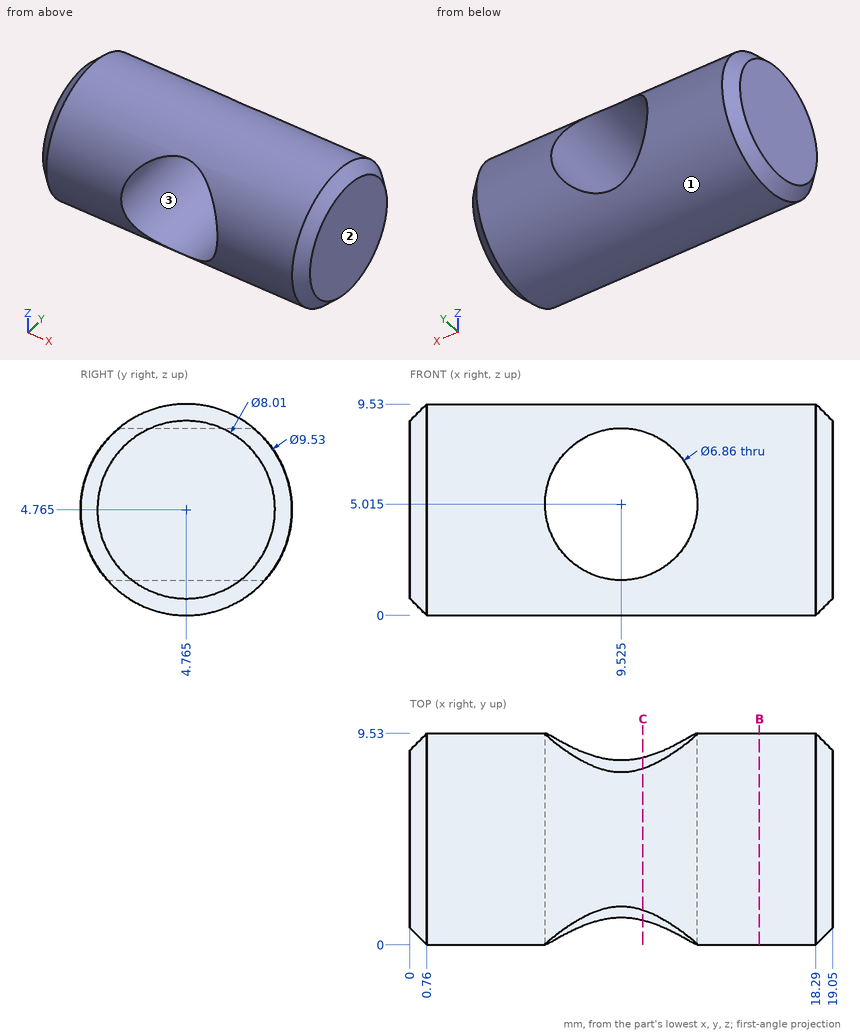
The drawing under review shows one solid part. Ordinate dimensions are in mm from its lowest x, y, z. Give positions to 0.01 mm unless a question says otherwise; leave off trailing zeros. Write each loop counter-clockwise with the first axis right and the second up, starting at its lowest first coordinate (ties: lowest second). Pieces come first, ordered by that corner, then holes. Notation, with made-up numbers: (-27, 30.25) -> (-9, 30.25) arc R32 ccw to (-9, 65.25) -> close; hole circle Ø2 at (-33.75, 53). An arc over 180 degrees is marked (long way). Answer in a Markdown table with one row per item.
(1) Consider section C-C (x = 10.5). State the section outline as (y, z) points (1 decimal).
Results:
| item | result |
|---|---|
| outline | (1.1, 1.7) arc R4.8 ccw to (8.4, 1.7) -> close; (1.6, 8.3) -> (8, 8.3) arc R4.8 ccw to start |
(2) Mouldability with a two-part tool opening along X and no side actions: class the marked faces 1, 2 and 3 as +X half, -X half, draft (parallel to the pull), parting line (faces both ways), or undercut.
Results:
| item | result |
|---|---|
| face 1 | draft |
| face 2 | +X half |
| face 3 | undercut |
(3) Clearance check with a flat-ended pin moving along its axis: pin 1 (1.5 mm diameter, centred on x = 2.5, y = 2.5, fed in from -Z). State where the tip first meets the part, or that it passes through.
Results:
| item | result |
|---|---|
| pin 1 | z = 0.25 |
(4) To check wall thickness, follow probe 1 along Z at (x, y) = (7.25, 8); probe 2 along X at (y, z) = (1.5, 7.25); probe 3 along Z at (x, y) = (11.75, 7). State the ranges of each line that lie inside material, in increasing order.
Results:
| item | result |
|---|---|
| probe 1 | 1.27 to 2.45, 7.58 to 8.26 |
| probe 2 | 0.1 to 6.92, 12.13 to 18.95 |
| probe 3 | 0.56 to 2.4, 7.63 to 8.97 |
(5) Consider section B-B (x = 15.75). State the section outline as (y, z) points (3 decimals), then the cut area to 3 significant figures.
Results:
| item | result |
|---|---|
| outline | circle Ø9.53 at (4.765, 4.765) |
| area | 71.3 mm2 |
